Geometry check sheet. Reference: the model listing, model coordinates, mm. Face numbers are marked on the shaded views. Round coordinates to 2 decimals unless told otherwise and drop trailing zeros. Order: outer loops, then holes, each group sorted by start corner. A loop starts at its lowest first (then second) coordinate and runs counter-clockwise, first axis right, second up.
```python
from build123d import *

# Parameters (mm, degrees)
F0_W     = 101
F0_H     = 101
F0_R     = 6
F1_DEPTH = 10
F0_W_2   = 119.4
F0_H_2   = 119.4
F2_DEPTH = 18
F3_R     = 2
F4_R     = 1


with BuildPart() as f1:
    # F0 (on Top) → F1 (new body)
    with BuildSketch(Plane.XY):
        Rectangle(F0_W, F0_H)
        Circle(F0_R, mode=Mode.SUBTRACT)
    extrude(amount=F1_DEPTH)

    # F0 (on Top) → F2 (join)
    with BuildSketch(Plane.XY):
        Rectangle(F0_W_2, F0_H_2)
        Rectangle(F0_W, F0_H, mode=Mode.SUBTRACT)
    extrude(amount=F2_DEPTH)

    # F3
    f3_edges = [f1.edges().sort_by_distance(p)[0] for p in [
        (-59.7, -59.7, 9),
        (59.7, -59.7, 9),
        (59.7, 59.7, 9),
        (-59.7, 59.7, 9),
    ]]
    fillet(f3_edges, radius=F3_R)

    # F4
    f4_edges = [f1.edges().sort_by_distance(p)[0] for p in [
        (59.7, 0, 0),
        (59.114214, -59.114214, 0),
        (59.114214, 59.114214, 0),
        (0, -59.7, 0),
        (0, 59.7, 0),
        (-59.114214, -59.114214, 0),
        (-59.114214, 59.114214, 0),
        (-59.7, 0, 0),
        (-6, 0, 0),
    ]]
    fillet(f4_edges, radius=F4_R)


solid = f1.part
```
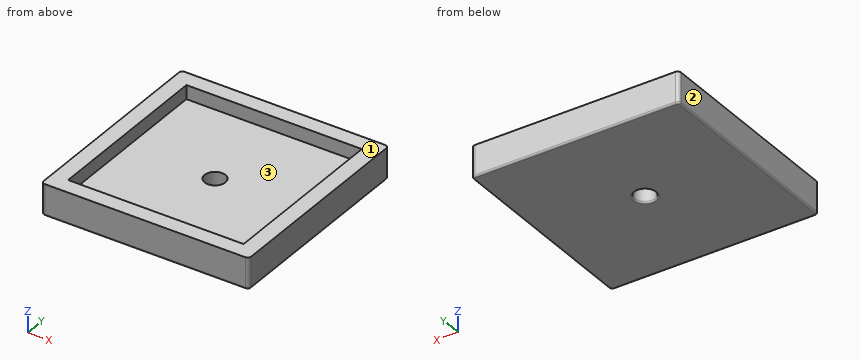
(1) Depth check by flat-ended pin: P1, Ø3, axis at x = 25, y = -45, coming from the +Z side; P2, Ø14, axis at x = 0, y = 0, coming from the -Z side. Enter the tip coordinate at first touch or a pass-through.
Returned:
P1: stops at z = 10
P2: stops at z = 0
(2) Sectioned sample at A-A, the plane x = 0. Record the cut outline in (y, z).
Returned:
outline: (-59.7, 1) arc R1 ccw to (-58.7, 0) - (-7, 0) arc R1 ccw to (-6, 1) - (-6, 10) - (-50.5, 10) - (-50.5, 18) - (-59.7, 18) - close; (6, 1) arc R1 ccw to (7, 0) - (58.7, 0) arc R1 ccw to (59.7, 1) - (59.7, 18) - (50.5, 18) - (50.5, 10) - (6, 10) - close
(3) Sectioned sample at C-C, the plane z = 11.75. Record the cut outline in (x, y).
Returned:
outline: (-59.7, -57.7) arc R2 ccw to (-57.7, -59.7) - (57.7, -59.7) arc R2 ccw to (59.7, -57.7) - (59.7, 57.7) arc R2 ccw to (57.7, 59.7) - (-57.7, 59.7) arc R2 ccw to (-59.7, 57.7) - close; hole (-50.5, -50.5) - (50.5, -50.5) - (50.5, 50.5) - (-50.5, 50.5) - close
(4) Material ranges on line 1 (Y direction, x = -49, z = 15.25); line 2 (Y direction, x = 0, z = 7.25), recorded low to high.
Returned:
line 1: y = -59.7 to -50.5, 50.5 to 59.7
line 2: y = -59.7 to -6, 6 to 59.7
(5) Draft check along X on the marked faces 1, 2 and 3. Enter one of: released by +X, released by -X, zero draft, split by the parting line, or undercut.
Returned:
face 1: zero draft
face 2: released by -X
face 3: undercut
(6) Sectioned sample at D-D, the plane y = -13.5. Record the cut outline in (x, z).
Returned:
outline: (-59.7, 1) arc R1 ccw to (-58.7, 0) - (58.7, 0) arc R1 ccw to (59.7, 1) - (59.7, 18) - (50.5, 18) - (50.5, 10) - (-50.5, 10) - (-50.5, 18) - (-59.7, 18) - close
